Source: CAD feature listing. Evaluate the final solid. Frame: model axes, mm. Face numbers are marked on the shaded views. Coordinates: 2 decimals unless noted, no trailing zeros. Loops run counter-clockwise (first coordinate to the right, second up) from the corner with the lowest first, then second, coordinate; pieces in that order, holes last.
Item 1: Line query: probe 1 along X at (y, z) = (5, -53.5); probe 2 along Z at (x, y) = (6, 3.5); probe 3 along X at (y, z) = (0.5, -32). Output: solid intervals per line, ascending.
Item 2: Pull-direction query (X, two-part tool) for the marked faces 1 and 2; classes: +X half, -X half, draft (parallel to the pull), parting line (faces both ways), or undercut.
Item 3: Section query D-D, the plane z = -75.5. Return the cut outline in (x, y), then the cut area to 3 significant figures.
Item 4: Section query C-C, the plane z = -9. Return the cut outline in (x, y), then the cut area to 3 significant figures.
Item 5: Pin query (flat end, axial travel): pin 1 Ø3 at (y, z) = (2.5, -44.5) entering from +X; pin 2 Ø3 at (y, z) = (7, -47.5) entering from -X; pin 3 Ø6 at (y, z) = (5.5, -70.5) entering from -X; pin 4 Ø2 at (x, y) = (149, 5) entering from -Z. Return the tip coordinate at first contact, or that it passes through.
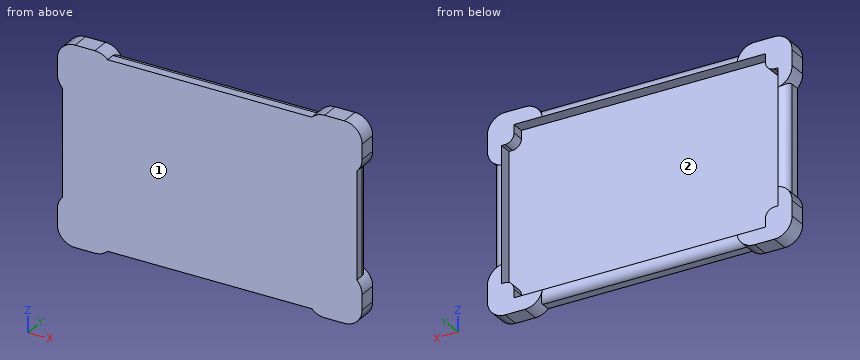
```python
from build123d import *

# Parameters (mm, degrees)
SKETCH7_W           = 165
SKETCH7_H           = 105
SKETCH7_W_2         = 145
SKETCH7_H_2         = 85
BOSS_EXTRUDE7_DEPTH = 10
SKETCH8_W           = 28.227937213
SKETCH8_H           = 25.640206581
BOSS_EXTRUDE8_DEPTH = 10
CUT_EXTRUDE4_DEPTH  = 7
FILLET2_R           = 10
FILLET3_R           = 5
FILLET6_R           = 5


# Some blends are built 0.0001 mm under size
with BuildPart() as part:
    # Sketch7 → Boss-Extrude7 (new body)
    # profile 1 of 2: a face of its own
    with BuildSketch(Plane(origin=(0, 0, 0), x_dir=(1, 0, 0), z_dir=(0, 1, 0))):
        with Locations((72.5, 42.5)):
            Rectangle(SKETCH7_W, SKETCH7_H)
        with Locations((72.5, 42.5)):
            Rectangle(SKETCH7_W_2, SKETCH7_H_2, mode=Mode.SUBTRACT)
    # profile 2 of 2: a face of its own
    with BuildSketch(Plane(origin=(0, 0, 0), x_dir=(1, 0, 0), z_dir=(0, 1, 0))):
        with Locations((72.5, 42.5)):
            Rectangle(SKETCH7_W_2, SKETCH7_H_2)
    extrude(amount=BOSS_EXTRUDE7_DEPTH)

    # Sketch8 → Boss-Extrude8 (add)
    with BuildSketch(Plane(origin=(0, 10, 0), x_dir=(1, 0, 0), z_dir=(0, 1, 0))):
        with Locations((1.113968607, -0.179896709)):
            Rectangle(SKETCH8_W, SKETCH8_H)
        with Locations((143.886031393, -0.179896709)):
            Rectangle(SKETCH8_W, SKETCH8_H)
        with Locations((143.886031393, 85.179896709)):
            Rectangle(SKETCH8_W, SKETCH8_H)
        with Locations((1.113968607, 85.179896709)):
            Rectangle(SKETCH8_W, SKETCH8_H)
    extrude(amount=-BOSS_EXTRUDE8_DEPTH)

    # Sketch10 → Cut-Extrude4 (cut)
    with BuildSketch(Plane(origin=(0, 10, 0), x_dir=(1, 0, 0), z_dir=(0, 1, 0))):
        Polygon((2, -5), (143, -5), (143, 4.63003775), (150, 4.63003775), (150, 80.36996225), (143, 80.36996225), (143, 90), (2, 90), (2, 80.36996225), (-5, 80.36996225), (-5, 4.63003775), (2, 4.63003775), align=None)
    extrude(amount=-CUT_EXTRUDE4_DEPTH, mode=Mode.SUBTRACT)

    # Fillet2
    # the kernel refuses this fillet: 10 mm, written as the material it takes off along each edge
    with BuildSketch(Plane(origin=(-13, 27.853571071, -72.359793419), x_dir=(1, 0, 0), z_dir=(0, -1, 0)), Plane(origin=(129.772062787, 27.853571071, -98), x_dir=(0, 0, 1), z_dir=(0, -1, 0)), Plane(origin=(158, 27.853571071, -12.640206581), x_dir=(-1, 0, 0), z_dir=(0, -1, 0)), Plane(origin=(15.227937213, 27.853571071, 13), x_dir=(0, 0, -1), z_dir=(0, -1, 0))) as fillet2_piece_1:
        with BuildLine():
            CenterArc((10, -7.141428429), FILLET2_R, 134.427004001, 45.572995999)
            Line((0, -7.141428429), (-0.2, -7.141428429))
            Line((-0.2, -7.141428429), (-0.2, 0))
            Line((-0.2, 0), (0, 0.2))
            ThreePointArc((0, 0.2), (1.5, 0.2), (2.86, 0.142828569))
            Line((2.86, 0.142828569), (3, 0))
        make_face()
    extrude(amount=45.707142143, mode=Mode.SUBTRACT)
    with BuildSketch(Plane(origin=(15.227937213, 27.853571071, -98), x_dir=(-1, 0, 0), z_dir=(0, -1, 0)), Plane(origin=(-13, 27.853571071, -12.640206581), x_dir=(0, 0, 1), z_dir=(0, -1, 0)), Plane(origin=(158, 27.853571071, -72.359793419), x_dir=(0, 0, -1), z_dir=(0, -1, 0)), Plane(origin=(129.772062787, 27.853571071, 13), x_dir=(1, 0, 0), z_dir=(0, -1, 0))) as fillet2_piece_2:
        with BuildLine():
            CenterArc((7.141428429, -10), FILLET2_R, 90, 45.572995999)
            Line((0, -3), (-0.142828569, -2.86))
            ThreePointArc((-0.142828569, -2.86), (-0.2, -1.5), (-0.2, 0))
            Line((-0.2, 0), (0, 0.2))
            Line((0, 0.2), (7.141428429, 0.2))
            Line((7.141428429, 0.2), (7.141428429, 0))
        make_face()
    extrude(amount=45.707142143, mode=Mode.SUBTRACT)
    with BuildSketch(Plane(origin=(-13, 35, -98), x_dir=(0, 0, 1), z_dir=(0, -1, 0)), Plane(origin=(158, 35, -98), x_dir=(-1, 0, 0), z_dir=(0, -1, 0)), Plane(origin=(158, 35, 13), x_dir=(0, 0, -1), z_dir=(0, -1, 0))) as fillet2_piece_3:
        with BuildLine():
            CenterArc((FILLET2_R, -FILLET2_R), FILLET2_R, 90, 90)
            Line((0, -FILLET2_R), (-FILLET2_R * 0.02, -FILLET2_R))
            Line((-FILLET2_R * 0.02, -FILLET2_R), (-FILLET2_R * 0.02, FILLET2_R * 0.02))
            Line((-FILLET2_R * 0.02, FILLET2_R * 0.02), (FILLET2_R, FILLET2_R * 0.02))
            Line((FILLET2_R, FILLET2_R * 0.02), (FILLET2_R, 0))
        make_face()
    extrude(amount=60, mode=Mode.SUBTRACT)
    with BuildSketch(Plane(origin=(-13, 35, 13), x_dir=(0, 0, -1), z_dir=(0, -1, 0))) as fillet2_piece_4:
        with BuildLine():
            CenterArc((FILLET2_R, FILLET2_R), FILLET2_R, 180, 90)
            Line((0, FILLET2_R), (-FILLET2_R * 0.02, FILLET2_R))
            Line((-FILLET2_R * 0.02, FILLET2_R), (-FILLET2_R * 0.02, -FILLET2_R * 0.02))
            Line((-FILLET2_R * 0.02, -FILLET2_R * 0.02), (FILLET2_R, -FILLET2_R * 0.02))
            Line((FILLET2_R, -FILLET2_R * 0.02), (FILLET2_R, 0))
        make_face()
    extrude(amount=60, mode=Mode.SUBTRACT)

    # Fillet3
    fillet3_edges = [part.edges().sort_by_distance(p)[0] for p in [
        (143, 6.5, -80.36996225),
        (143, 6.5, -4.63003775),
        (2, 6.5, -4.63003775),
        (2, 6.5, -80.36996225),
    ]]
    fillet(fillet3_edges, radius=FILLET3_R)

    # Fillet6
    fillet6_edges = [part.edges().sort_by_distance(p)[0] for p in [
        (72.5, 10, -95),
        (155, 10, -42.5),
        (72.5, 10, 10),
        (-10, 10, -42.5),
    ]]
    fillet(fillet6_edges, radius=FILLET6_R - 0.0001)  # a hair under: the kernel refuses the full size


solid = part.part
```
Verdict:
1. probe 1: x = -10 to -5, 150 to 155
1. probe 2: z = -98 to -90, 5 to 13
1. probe 3: x = -10 to 155
2. face 1: draft
2. face 2: undercut
3. outline: (-12.16, 0) - (157.16, 0) - (157.16, 10) - (150, 10) - (150, 3) - (-5, 3) - (-5, 10) - (-12.16, 10) - close
3. area: 608 mm2
4. outline: (-12.37, 0) - (157.37, 0) - (157.37, 10) - (150, 10) - (150, 3) - (-5, 3) - (-5, 10) - (-12.37, 10) - close
4. area: 612 mm2
5. pin 1: stops at x = 155
5. pin 2: stops at x = -9.97
5. pin 3: stops at x = -11
5. pin 4: stops at z = -98
